Source: CAD feature listing. Evaluate the final solid. Frame: model axes, mm. A direction names the side the tool comes from. Round coordinates to 2 decimals unless told otherwise and drop trailing zeros. Order: outer loops, then holes, each group sorted by start corner. A loop starts at its lowest first (then second) coordinate and runs counter-clockwise, first axis right, second up. Notation, with made-up numbers: (0, 66) -> (9, 66) arc R21 ccw to (9, 95) -> close; hole circle Ø3 at (32.25, 77.5). An arc over 180 degrees is marked (long way). Answer as CSV lines item,"result". Start each with the question number.
(1) Section query A-A (y = 1). Output: boundary loops of the cut face in (x, z).
(2) Section query B-B (z = 1.25). Output: boundary loops of the cut face in (x, y), plus the area to 3 significant figures.
(3) Pull-direction query (X, two-part tool) for faces 4 (the flat face through (26, 3.81, 3)), 5 (the flat face through (3, 0, 3)), 6 (the flat face through (50.8, 3, 3)); classes: +X half, -X half, draft (parallel to the pull), parting line (faces both ways), or undercut.
(4) Set-up query: faces 1 (the cylindrical face through (46.11, 3.65, 6.98)), 2 (the flat face through (6.35, 2, 3)), 3 (the flat face through (48, 3, 7.62)). Return all of +Z, -Z, +X, -X, +Y, -Y with unobstructed straight access to the full face (end or side cutting, diameter ignored); none if empty.
(5) Section query D-D (y = 5.5). Output: boundary loops of the cut face in (x, z).
(6) Line query: line 1 along X through (y, z) = (1, 2.25); line 2 along Y through (x, z) = (18, 4.25); line 3 along Z through (x, y) = (29.5, 4.5). Output: solid intervals per line, ascending. Write a range as from..to.
(7) Contact query for a flat-ended pin moving along its axis: P1, Ø1.9, axis at x = 34, y = 3.5, coming from the +Z side. Output: stop coordinate, or through.
(8) Section query C-C (x = 14.5). Output: boundary loops of the cut face in (y, z).
```python
from build123d import *

# Parameters (mm, degrees)
SKETCH1_W           = 6.35
SKETCH1_H           = 6.35
SKETCH1_W_2         = 19.05
SKETCH1_H_2         = 2.54
BOSS_EXTRUDE1_DEPTH = 6.35
SKETCH2_R           = 1.5875
BOSS_EXTRUDE2_DEPTH = 1.27


with BuildPart() as part:
    # Sketch1 → Boss-Extrude1 (new body)
    with BuildSketch(Plane.XY):
        with Locations((3.175, 3.175)):
            Rectangle(SKETCH1_W, SKETCH1_H)
        with Locations((15.875, 5.08)):
            Rectangle(SKETCH1_W_2, SKETCH1_H_2)
    boss_extrude1 = extrude(amount=BOSS_EXTRUDE1_DEPTH)

    # Sketch2 → Boss-Extrude2 (add)
    with BuildSketch(Plane.XY.offset(6.35)):
        with Locations((3.175, 3.175)):
            Circle(SKETCH2_R)
    boss_extrude2 = extrude(amount=BOSS_EXTRUDE2_DEPTH)

    # Mirror1: Boss-Extrude1, Boss-Extrude2 across plane
    add(boss_extrude1.mirror(Plane(origin=(25.4, 0, 6.35), x_dir=(0, 0, 1), z_dir=(1, 0, 0))))
    add(boss_extrude2.mirror(Plane(origin=(25.4, 0, 6.35), x_dir=(0, 0, 1), z_dir=(1, 0, 0))))


solid = part.part
```
Answer block:
1,outline,"(0, 0) -> (6.35, 0) -> (6.35, 6.35) -> (0, 6.35) -> close; (44.45, 0) -> (50.8, 0) -> (50.8, 6.35) -> (44.45, 6.35) -> close"
2,outline,"(0, 0) -> (6.35, 0) -> (6.35, 3.81) -> (44.45, 3.81) -> (44.45, 0) -> (50.8, 0) -> (50.8, 6.35) -> (0, 6.35) -> close"
2,area,"177 mm2"
3,face 4,"undercut"
3,face 5,"draft"
3,face 6,"+X half"
4,face 1,"+Z"
4,face 2,"+Z, -Z, -Y"
4,face 3,"+Z, +X, -X, +Y, -Y"
5,outline,"(0, 0) -> (50.8, 0) -> (50.8, 6.35) -> (0, 6.35) -> close"
6,line 1,"0..6.35, 44.45..50.8"
6,line 2,"3.81..6.35"
6,line 3,"0..6.35"
7,P1,"z = 6.35"
8,outline,"(3.81, 0) -> (6.35, 0) -> (6.35, 6.35) -> (3.81, 6.35) -> close"
